Autodesk Inventor part; units mm, degrees
ref_plane "YZ Plane" through (0, 0, 0) normal (1, 0, 0) x (0, 1, 0)
ref_plane "XZ Plane" through (0, 0, 0) normal (0, 1, 0) x (-1, 0, 0)
ref_plane "XY Plane" through (0, 0, 0) normal (0, 0, 1) x (1, 0, 0)
sketch "Sketch1" plane through (0, 0, 0) normal (0, 1, 0) x (-1, 0, 0)
  circle A0 centre (0, 0) radius 100
  dimension "d0" = 200
extrude "Extrusion1" add sketch "Sketch1" along normal blind 75
chamfer "Chamfer1" distance 5 angle 45 2 edges at (100, 75, 0) (100, 0, 0)
sketch "Sketch2" plane through (0, 75, 0) normal (0, 1, 0) x (1, 0, 0)
  circle A0 centre (0, 0) radius 10
  dimension "d6" = 20
extrude "Extrusion2" cut sketch "Sketch2" against normal blind 75
chamfer "Chamfer2" distance 5 angle 45 2 edges at (-10, 75, 0) (-10, 0, 0)
properties part number "Peso"
The model under review builds one solid part; all positions refer to its coordinate system, in mm. Give positions to 0.01 mm unless a question says otherwise; leave off trailing zeros. Order: outer loops, then holes, each group sorted by start corner. A loop starts at its lowest first (then second) coordinate and runs counter-clockwise, first axis right, second up. Notation, with made-up numbers: (62.5, -22) - (111.5, -22) arc R11 cw to (111.5, -14) - close; hole circle Ø7 at (33, 74). An arc over 180 degrees is marked (long way). Use CSV: the item, a comma, the result in double quotes. Start each with the question number.
Q1. We need section C-C, the plane y = 39. Write out the cut boundary in (x, z).
Q2. The part is to be moulded in two halves that separate along Z. For faces 1 (the flat face through (-20, 75, 1)), 2 (the conical face through (20.662, 0.313, -93.046)), 3 (the conical face through (-2.236, 4.687, -10.068)), say which applies: +Z half, -Z half, draft (parallel to the pull), parting line (faces both ways), or undercut.
Q3. To check wall thickness, follow line 1 along Z through (x, y) = (0, 38); line 2 along X through (y, z) = (32, -9); line 3 along X through (y, z) = (9.5, 5.5). State the ranges of each line that lie inside material, in increasing order. Write a range as [from, to].
Q4. We need section B-B, the plane x = 0. Write out the cut boundary in (y, z).
Q5. We need section A-A, the plane z = 0. Write out the cut boundary in (x, y), and give its area (3 significant figures).
Q6. Clearance check with flat-ended pins moving along their axes: pin 1 Ø1.5 at (y, z) = (64, 73) entering from +X; pin 2 Ø12 at (y, z) = (9.5, -19) entering from +X; pin 3 Ø1.5 at (y, z) = (29.5, -50) entering from +X. State where each tip first meets the part, or that it passes through.
Outcome:
1,outline,"circle Ø200 at (0, 0); hole circle Ø20 at (0, 0)"
2,face 1,"draft"
2,face 2,"parting line"
2,face 3,"undercut"
3,line 1,"z = [-100, -10], [10, 100]"
3,line 2,"x = [-99.59, -4.36], [4.36, 99.59]"
3,line 3,"x = [-99.85, -8.35], [8.35, 99.85]"
4,outline,"(0, -95) - (5, -100) - (70, -100) - (75, -95) - (75, -15) - (70, -10) - (5, -10) - (0, -15) - close; (0, 15) - (5, 10) - (70, 10) - (75, 15) - (75, 95) - (70, 100) - (5, 100) - (0, 95) - close"
5,outline,"(-100, 5) - (-95, 0) - (-15, 0) - (-10, 5) - (-10, 70) - (-15, 75) - (-95, 75) - (-100, 70) - close; (10, 5) - (15, 0) - (95, 0) - (100, 5) - (100, 70) - (95, 75) - (15, 75) - (10, 70) - close"
5,area,"13,400 mm^2"
6,pin 1,"stops at x = 69.14"
6,pin 2,"stops at x = 99.15"
6,pin 3,"stops at x = 87.03"
